Verification items for the finished model (mm, model axes). Coordinates: 2 decimals unless noted, no trailing zeros. Write each loop counter-clockwise with the first axis right and the second up, starting at its lowest first coordinate (ties: lowest second). Pieces come first, ordered by that corner, then holes. Notation, with made-up numbers: (5, 10.5) - (59, 10.5) arc R7 ccw to (59, 23.5) - close; hole circle Ø9 at (30, 16.25). An arc over 180 degrees is marked (long way). Use one line per item in the form item = value. Start each with the question number.
(1) Sectioned sample at B-B (y = -99). Record the cut outline in (x, z).
(2) Sectioned sample at A-A (x = 0). Record the cut outline in (y, z).
(3) Sectioned sample at C-C (z = 20.75). Record the cut outline in (x, y).
(4) Gauge pin test, flat ends, axial feed: pin 1 Ø5 at (y, z) = (-63.5, 3.5) entering from -X; pin 2 Ø5 at (x, z) = (-19, 10) entering from +Y; pin 3 Ø2 at (x, z) = (-83, 2.5) entering from +Y (3 decimals). Record the tip position at first contact, or that the pin passes through.
(5) Material ranges on line 1 (Y direction, x = 122.5, z = 17.25); line 2 (X direction, y = -105, z = 11.5); line 3 (X direction, y = 4, z = 2.25), recorded low to high. Write a range as [from, to].
(6) Mould release check, pull along Y, two halves, no side actions. Record for faces 1 (the cylindrical face through (1.38, -6.2, 12.52)), 2 (the cylindrical face through (1.19, 76.21, 12.52)), 3 (the cylindrical face through (-69.96, -120.92, 12.52)): released by +Y, released by -Y, zero draft, split by the parting line, or undercut.
(7) Sectioned sample at D-D (x = 88). Record the cut outline in (y, z), and give its area (3 significant figures).
from build123d import *

# Parameters (mm, degrees)
F2_DEPTH = 25.4
F4_D     = 12.7
F4_DEPTH = 127


with BuildPart() as f2:
    # F0 (on Top) → F2 (new body)
    with BuildSketch(Plane.XY):
        with BuildLine():
            ThreePointArc((139.404567, -9.080571), (139.626122, -4.542688), (139.7, 0))
            ThreePointArc((139.7, 0), (139.626122, 4.542688), (139.404567, 9.080571))
            ThreePointArc((139.404567, 9.080571), (65.991136, 38.1), (77.566289, 116.187611))
            ThreePointArc((77.566289, 116.187611), (69.85, 120.983749), (61.838278, 125.268182))
            ThreePointArc((61.838278, 125.268182), (0, 76.2), (-61.838278, 125.268182))
            ThreePointArc((-61.838278, 125.268182), (-69.85, 120.983749), (-77.566289, 116.187611))
            ThreePointArc((-77.566289, 116.187611), (-62.720301, 95.101151), (-57.483749, 69.85))
            ThreePointArc((-57.483749, 69.85), (-83.151699, 18.850138), (-139.404567, 9.080571))
            ThreePointArc((-139.404567, 9.080571), (-139.7, 0), (-139.404567, -9.080571))
            ThreePointArc((-139.404567, -9.080571), (-83.151699, -18.850138), (-57.483749, -69.85))
            ThreePointArc((-57.483749, -69.85), (-62.720301, -95.101151), (-77.566289, -116.187611))
            ThreePointArc((-77.566289, -116.187611), (-69.85, -120.983749), (-61.838278, -125.268182))
            ThreePointArc((-61.838278, -125.268182), (0, -76.2), (61.838278, -125.268182))
            ThreePointArc((61.838278, -125.268182), (69.85, -120.983749), (77.566289, -116.187611))
            ThreePointArc((77.566289, -116.187611), (65.991136, -38.1), (139.404567, -9.080571))
        make_face()
    extrude(amount=F2_DEPTH)

    # F4
    with Locations(Plane.XY.offset(25.4)):
        with Locations((0, 0)):
            Hole(F4_D / 2, depth=F4_DEPTH)


solid = f2.part
Answers below:
q1.outline = (-64.57, 0) - (-48.74, 0) - (-48.74, 25.4) - (-64.57, 25.4) - close; (48.74, 0) - (64.57, 0) - (64.57, 25.4) - (48.74, 25.4) - close
q2.outline = (-76.2, 0) - (-6.35, 0) - (-6.35, 25.4) - (-76.2, 25.4) - close; (6.35, 0) - (76.2, 0) - (76.2, 25.4) - (6.35, 25.4) - close
q3.outline = (-139.4, -9.08) arc R63.5 cw to (-57.48, -69.85) arc R63.5 cw to (-77.57, -116.19) arc R139.7 ccw to (-61.84, -125.27) arc R63.5 cw to (61.84, -125.27) arc R139.7 ccw to (77.57, -116.19) arc R63.5 cw to (139.4, -9.08) arc R139.7 ccw to (139.7, 0) arc R139.7 ccw to (139.4, 9.08) arc R63.5 cw to (77.57, 116.19) arc R139.7 ccw to (61.84, 125.27) arc R63.5 cw to (-61.84, 125.27) arc R139.7 ccw to (-77.57, 116.19) arc R63.5 cw to (-57.48, 69.85) arc R63.5 cw to (-139.4, 9.08) arc R139.7 ccw to start; hole circle Ø12.7 at (0, 0)
q4.pin_1 = -58.1
q4.pin_2 = 79.95
q4.pin_3 = 19.725
q5.line_1 = [-6.37, 6.37]
q5.line_2 = [-68.1, -53.18], [53.18, 68.1]
q5.line_3 = [-139.64, -4.93], [4.93, 139.64]
q6.face_1 = undercut
q6.face_2 = released by +Y
q6.face_3 = released by -Y
q7.outline = (-15.59, 0) - (15.59, 0) - (15.59, 25.4) - (-15.59, 25.4) - close
q7.area = 792 mm2
